Input: part model. Units: mm. Frame: model coordinates. Round coordinates to 2 decimals unless told otherwise and drop trailing zeros. Loops run counter-clockwise (first coordinate to the right, second up) from the corner with the lowest first, then second, coordinate; pieces in that order, holes last. Notation, with made-up numbers: (36.5, -28.5) -> (91.5, -28.5) arc R35 cw to (91.5, 7.5) -> close; hole circle Ø3 at (-6.75, 13). An arc over 180 degrees is marked (long way). One line per question, with ' | ' between items. Start each with the question number.
Q1. Cut plane D-D on z = -0.6. Return loops of the section in (x, y).
Q2. Cut plane C-C on y = 8. Return loops of the section in (x, z), and give its area (3 significant figures).
Q3. Contact query for flat-ended pins moving along their axis: P1, Ø1, axis at x = -1, y = 4, coming from the -Z side; P2, Ø1, axis at x = -1, y = 5, coming from the +Z side; P3, Ø1.5, axis at x = -1, y = 7, coming from the +Z side. Output: stop coordinate, or through.
Q4. Material intervals for L1, parallel to Y at x = -0.7, z = 0.1; L2, parallel to Y at x = 0.6, z = -0.85; L3, parallel to Z at x = -0.1, y = 7.25, sorted ascending.
Q5. Cut plane B-B on x = 1.1. Return loops of the section in (y, z).
Q6. Cut plane A-A on z = 0. Return loops of the section in (x, y), and give its area (3 significant figures).
from build123d import *

# Parameters (mm, degrees)
SKETCH1_R               = 1.25
BOSS_EXTRUDE1_DEPTH     = 6
SKETCH2_R               = 1.25
BOSS_EXTRUDE2_DEPTH     = 5
SKETCH3_R               = 1.25
BOSS_EXTRUDE3_DEPTH     = 5
CUT_EXTRUDE1_DEPTH      = 2.25
CUT_EXTRUDE1_DEPTH_BACK = 2.25


with BuildPart() as part:
    # Sketch1 → Boss-Extrude1 (new body)
    with BuildSketch(Plane(origin=(0, 0, 0), x_dir=(1, 0, 0), z_dir=(0, 1, 0))):
        Circle(SKETCH1_R)
    extrude(amount=BOSS_EXTRUDE1_DEPTH)

    # Sketch2 → Boss-Extrude2 (add)
    with BuildSketch(Plane.XZ):
        Circle(SKETCH2_R)
    extrude(amount=BOSS_EXTRUDE2_DEPTH)

    # Sketch3 → Boss-Extrude3 (add)
    with BuildSketch(Plane(origin=(0, 6, 0), x_dir=(1, 0, 0), z_dir=(0, 1, 0))):
        Circle(SKETCH3_R)
    extrude(amount=BOSS_EXTRUDE3_DEPTH)

    # Sketch4 → Cut-Extrude1 (cut, two sides)
    with BuildSketch(Plane.XY) as cut_extrude1_sk:
        Polygon((0.524763121, 9), (1.25, 9.725236879), (1.25, 8.274763121), align=None)
        Polygon((-0.524763121, 9), (-1.25, 8.274763121), (-1.25, 9.725236879), align=None)
        Polygon((-0.524763121, -3), (-1.25, -3.725236879), (-1.25, -2.274763121), align=None)
        Polygon((0.524763121, -3), (1.25, -2.274763121), (1.25, -3.725236879), align=None)
    extrude(amount=CUT_EXTRUDE1_DEPTH, mode=Mode.SUBTRACT)
    extrude(cut_extrude1_sk.sketch, amount=-CUT_EXTRUDE1_DEPTH_BACK, mode=Mode.SUBTRACT)


solid = part.part
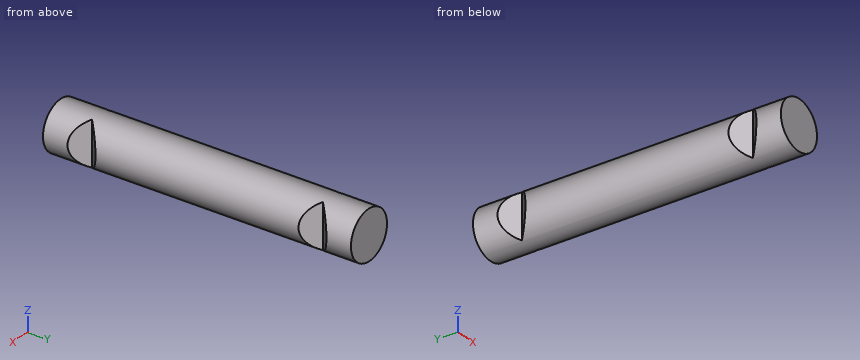
Results:
1) outline: (-1.1, -5) -> (1.1, -5) -> (1.1, -3.57) -> (0.52, -3) -> (1.1, -2.43) -> (1.1, 8.43) -> (0.52, 9) -> (1.1, 9.57) -> (1.1, 11) -> (-1.1, 11) -> (-1.1, 9.57) -> (-0.52, 9) -> (-1.1, 8.43) -> (-1.1, -2.43) -> (-0.52, -3) -> (-1.1, -3.57) -> close
2) outline: circle Ø2.5 at (0, 0) | area: 4.91 mm^2
3) P1: z = -1.15 | P2: z = 1.15 | P3: z = 1.22
4) L1: -5 to -3.18, -2.82 to 8.82, 9.18 to 11 | L2: -5 to -3.08, -2.92 to 8.92, 9.08 to 11 | L3: -1.25 to 1.25
5) outline: (-5, -0.59) -> (-3.58, -0.59) -> (-3.58, 0.59) -> (-5, 0.59) -> close; (-2.42, -0.59) -> (8.42, -0.59) -> (8.42, 0.59) -> (-2.42, 0.59) -> close; (9.58, -0.59) -> (11, -0.59) -> (11, 0.59) -> (9.58, 0.59) -> close
6) outline: (-1.25, -5) -> (1.25, -5) -> (1.25, -3.73) -> (0.52, -3) -> (1.25, -2.27) -> (1.25, 8.27) -> (0.52, 9) -> (1.25, 9.73) -> (1.25, 11) -> (-1.25, 11) -> (-1.25, 9.73) -> (-0.52, 9) -> (-1.25, 8.27) -> (-1.25, -2.27) -> (-0.52, -3) -> (-1.25, -3.73) -> close | area: 37.9 mm^2
